```python
from build123d import *

# Parameters (mm, degrees)
F0_W     = 457.2
F0_H     = 330.2
F1_DEPTH = 101.6
F2_W     = 412.75
F2_H     = 292.1
F3_DEPTH = 88.9
F4_R     = 25.4
F4_R_2   = 19.05
F5_DEPTH = 12.7
F6_R     = 36.615216
F7_DEPTH = 127


with BuildPart() as f1:
    # F0 (on Front) → F1 (new body)
    with BuildSketch(Plane.XZ):
        with Locations((0.697471, -6.70637)):
            Rectangle(F0_W, F0_H)
    extrude(amount=F1_DEPTH)

    # F2 (on face) → F3 (cut)
    with BuildSketch(Plane(origin=(0, 0, 0), x_dir=(-1, 0, 0), z_dir=(0, 1, 0))):
        with Locations((0, -9.88137)):
            Rectangle(F2_W, F2_H)
    extrude(amount=-F3_DEPTH, mode=Mode.SUBTRACT)

    # F4 (on face) → F5 (cut, through all)
    with BuildSketch(Plane.XZ.offset(101.6)):
        with Locations((-35.404028, 3.124894)):
            Circle(F4_R)
        with Locations((-110.152276, 2.381926)):
            Circle(F4_R)
        with Locations((-35.554084, 59.31631)):
            Circle(F4_R_2)
        with Locations((-73.534027, -57.157114)):
            Circle(F4_R_2)
        with Locations((36.530149, 59.164049)):
            Circle(F4_R_2)
        with Locations((110.887155, 1.915031)):
            Circle(F4_R)
        with Locations((36.142713, 2.973768)):
            Circle(F4_R)
        with Locations((74.928969, -57.157114)):
            Circle(F4_R_2)
    extrude(amount=-F5_DEPTH, mode=Mode.SUBTRACT)

    # F6 (on face) → F7 (join)
    with BuildSketch(Plane.YZ.offset(229.297471)):
        with Locations((-57.18055, 10.966711)):
            Circle(F6_R)
    extrude(amount=F7_DEPTH)


solid = f1.part
```
Check sheet for the modelled part. Datum: model origin and axes. Units: mm. A direction names the side the tool comes from. Give positions to 0.01 mm unless a question says otherwise; leave off trailing zeros. Order: outer loops, then holes, each group sorted by start corner. A loop starts at its lowest first (then second) coordinate and runs counter-clockwise, first axis right, second up. Notation, with made-up numbers: M 43.25,44.25 L 61.25,44.25 A22 ccw 61.25,53.25 Z; hole C 9,37.25 d5. An arc over 180 degrees is marked long. Answer in a Markdown table with one row per item. Add a question column.
Q1. Thickness scan on L1, parallel to X at y = -63, z = -132 (3 decimals); L2, parallel to Z at x = -111, y = -55; L3, parallel to Y at x = 33.5, z = -77. Record the ranges inside material, lowest first.
Q2. Sectioned sample at B-B, the plane x = 101.5. Record the boundary of the cut face in (y, z).
Q3. Gauge pin test, flat ends, axial feed: pin 1 Ø1 at (x, z) = (-43.5, -76.5) entering from +Y; pin 2 Ø8 at (y, z) = (-56.5, 113.5) entering from +X; pin 3 Ø8 at (x, z) = (228.5, -6) entering from +Y. Record the tip position at first contact, or that the pin passes through.
Q4. Sectioned sample at C-C, the plane z = -119.5. Record the boundary of the cut face in (x, y) (3 decimals).
Q5. Sectioned sample at D-D, the plane x = -38.5. Record the boundary of the cut face in (y, z), and give its area (3 significant figures).
Q6. Sectioned sample at A-A, the plane y = -82.5. Record the boundary of the cut face in (x, z) (3 decimals), and give its area (3 significant figures).
Q7. Access from +Z, -Z, +X, -X, +Y, -Y to the whole of each face (thin tool, end or side, straight path). Record for faces 1 (the cylindrical face through (-11.94, -95.34, -6.6)), 2 (the cylindrical face through (291.91, -93.76, 12.58)), 3 (the flat face through (206.375, -44, -12)).
Q8. Release check for a two-part mould opening along X. For faces 4 (the cylindrical face through (55.9, -95.3, -56.3)), 5 (the flat face through (229.297, -16, -9)), 6 (the flat face through (-3, -50, -171.806)) record: released by +X, released by -X, zero draft, split by the parting line, or undercut.
Verdict:
| question | item | result |
|---|---|---|
| 1 | L1 | -227.903 to -206.375, 206.375 to 229.297 |
| 1 | L2 | -171.81 to -155.93, 136.17 to 158.39 |
| 1 | L3 | -101.6 to -88.9 |
| 2 | outline | M -101.6,-171.81 L 0,-171.81 L 0,-155.93 L -88.9,-155.93 L -88.9,-21.69 L -101.6,-21.69 Z; M -101.6,25.52 L -88.9,25.52 L -88.9,136.17 L 0,136.17 L 0,158.39 L -101.6,158.39 Z |
| 3 | pin 1 | y = -88.9 |
| 3 | pin 2 | x = 229.3 |
| 3 | pin 3 | y = 0 |
| 4 | outline | M -227.903,-101.6 L 229.297,-101.6 L 229.297,0 L 206.375,0 L 206.375,-88.9 L -206.375,-88.9 L -206.375,0 L -227.903,0 Z |
| 5 | outline | M -101.6,-171.81 L 0,-171.81 L 0,-155.93 L -88.9,-155.93 L -88.9,-22.09 L -101.6,-22.09 Z; M -101.6,28.34 L -88.9,28.34 L -88.9,40.5 L -101.6,40.5 Z; M -101.6,78.14 L -88.9,78.14 L -88.9,136.17 L 0,136.17 L 0,158.39 L -101.6,158.39 Z |
| 5 | area | 6,460 mm² |
| 6 | outline | M -227.903,-171.806 L 229.297,-171.806 L 229.297,-15.483 L 356.297,-15.483 L 356.297,37.417 L 229.297,37.417 L 229.297,158.394 L -227.903,158.394 Z; hole M -206.375,-155.931 L 206.375,-155.931 L 206.375,136.169 L -206.375,136.169 Z |
| 6 | area | 37,100 mm² |
| 7 | face 1 | +Y, -Y |
| 7 | face 2 | +X |
| 7 | face 3 | +Y |
| 8 | face 4 | undercut |
| 8 | face 5 | released by +X |
| 8 | face 6 | zero draft |
